Here's the drawing with two shaded views (mm, measured from the low corner). I have some questions. A direction names the side the tool comes from. Coordinates: 2 decimals unless noted, no trailing zeros. Write each loop counter-clockwise with the first axis right and the second up, starting at its lowest first coordinate (ties: lowest second). Pieces come first, ordered by that corner, then holes. Notation, with made-up numbers: (-39, 53.5) - (19, 53.5) arc R13 ccw to (19, 73.5) - close; hole circle Ø7 at (8, 7.5). An arc over 180 degrees is marked (long way). Answer in a Markdown table with one row per item. Add a question column.
Item 1: I'm going to push flat-ended pins straight in: pin 1 (2 mm diameter, centred on x = 23, z = 25.5, fed in from -Y); pin 2 (1 mm diameter, centred on y = 12.5, z = 12.5, fed in from +X); pin 3 (2 mm diameter, centred on x = 27.5, y = 9, fed in from +Z); pin 4 (6.5 mm diameter, centred on y = 6, z = 20.5, fed in from +X). Where does each tip first touch, or does it pass through?
Item 2: If I drill on probe 1 along X at (y, z) = (11, 27.5); probe 2 along X at (y, z) = (6.5, 12.5), over which ranges is the centre line in solid material (lowest first)? Write a range as from..to.
Item 3: We'd pull the mould along Z, two halves only. Please class the marked faces 5, 6, 7 and 8: +Z half, -Z half, draft (parallel to the pull), parting line (faces both ways), or undercut.
Item 4: Imagine slicing it at C-C (y = 8.75). Please give me the cut outline in (x, z).
Item 5: Imagine slicing it at D-D (y = 1). Please give me the cut outline in (x, z).
Item 6: Imagine slicing it at A-A (x = 14). Please give me the cut outline in (y, z).
Item 7: Imagine slicing it at B-B (z = 28). Please give me the cut outline in (x, y), plus the area to 3 significant figures.
Item 8: Which directions (+Z, -Z, +X, -X, +Y, -Y) give clear straight access to the entire face, cutting with the end or side of a thin tool? Please do the marked faces 1, 2, 3 and 4.
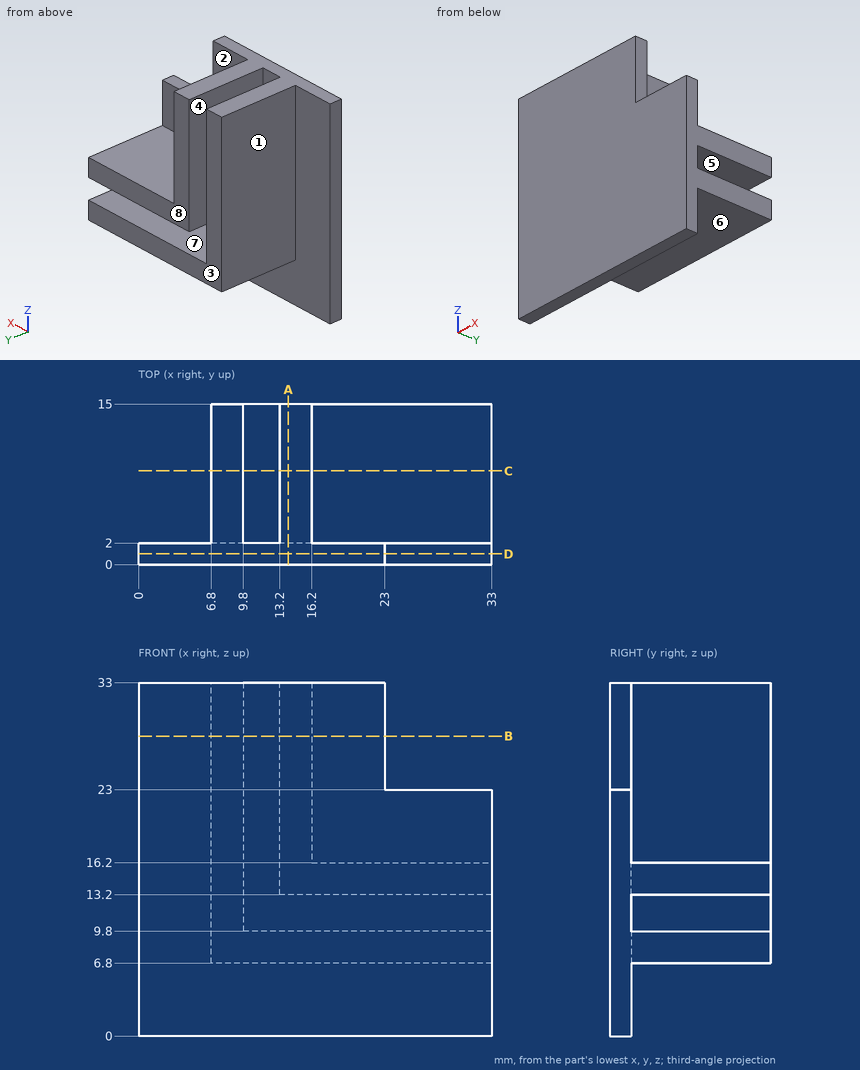
Here are the results:
| question | item | result |
|---|---|---|
| 1 | pin 1 | stops at y = 0 |
| 1 | pin 2 | stops at x = 9.8 |
| 1 | pin 3 | stops at z = 16.2 |
| 1 | pin 4 | stops at x = 16.2 |
| 2 | probe 1 | x = 6.8..9.8, 13.2..16.2 |
| 2 | probe 2 | x = 6.8..9.8 |
| 3 | face 5 | undercut |
| 3 | face 6 | -Z half |
| 3 | face 7 | undercut |
| 3 | face 8 | draft |
| 4 | outline | (6.8, 6.8) - (33, 6.8) - (33, 9.8) - (9.8, 9.8) - (9.8, 33) - (6.8, 33) - close; (13.2, 13.2) - (33, 13.2) - (33, 16.2) - (16.2, 16.2) - (16.2, 33) - (13.2, 33) - close |
| 5 | outline | (0, 0) - (33, 0) - (33, 23) - (23, 23) - (23, 33) - (0, 33) - close |
| 6 | outline | (0, 0) - (2, 0) - (2, 6.8) - (15, 6.8) - (15, 9.8) - (2, 9.8) - (2, 13.2) - (15, 13.2) - (15, 33) - (0, 33) - close |
| 7 | outline | (0, 0) - (23, 0) - (23, 2) - (16.2, 2) - (16.2, 15) - (13.2, 15) - (13.2, 2) - (9.8, 2) - (9.8, 15) - (6.8, 15) - (6.8, 2) - (0, 2) - close |
| 7 | area | 124 mm2 |
| 8 | face 1 | +Z, -Z, -X, +Y |
| 8 | face 2 | +Z, +X, +Y |
| 8 | face 3 | +Z, -Z, +X, -X, +Y |
| 8 | face 4 | +Z, +Y |
